CAD build for the part. Positions are in the model's coordinates, mm. A direction names the side the tool comes from. Coordinates: 2 decimals unless noted, no trailing zeros. Order: outer loops, then holes, each group sorted by start corner. A loop starts at its lowest first (then second) coordinate and runs counter-clockwise, first axis right, second up. Notation, with made-up numbers: M -27.75,26 L -7.75,26 A3 ccw -7.75,31 Z; hole C 54.5,17 d4. An arc over 180 degrees is marked long. Write item = value, one per line.
from build123d import *

# Parameters (mm, degrees)
F0_W     = 28.2
F0_H     = 28.2
F0_R     = 11.4
F0_R_2   = 2.25
F1_DEPTH = 28.2
F2_DEPTH = 2
F3_R     = 2.5
F5_D     = 2.5
F5_DEPTH = 5
F5_TIP   = 0.7510757738


with BuildPart() as f1:
    # F0 (on Top) → F1 (new body)
    with BuildSketch(Plane.XY):
        Rectangle(F0_W, F0_H)
        Circle(F0_R, mode=Mode.SUBTRACT)
        Circle(F0_R)
        Circle(F0_R_2, mode=Mode.SUBTRACT)
    extrude(amount=-F1_DEPTH)

    # F0 (on Top) → F2 (join)
    with BuildSketch(Plane.XY):
        Circle(F0_R)
        Circle(F0_R_2, mode=Mode.SUBTRACT)
    extrude(amount=F2_DEPTH)

    # F3
    f3_edges = [f1.edges().sort_by_distance(p)[0] for p in [
        (-14.1, -14.1, -14.1),
        (14.1, -14.1, -14.1),
        (-14.1, 14.1, -14.1),
        (14.1, 14.1, -14.1),
    ]]
    fillet(f3_edges, radius=F3_R)

    # F5
    with Locations(Plane.XY):
        with Locations((-11.5, 11.5), (11.5, 11.5), (11.5, -11.5), (-11.5, -11.5)):
            Hole(F5_D / 2, depth=F5_DEPTH)
            with Locations((0, 0, -(F5_DEPTH + F5_TIP / 2))):  # 118° drill point
                Cone(0, F5_D / 2, F5_TIP, mode=Mode.SUBTRACT)


solid = f1.part
(1) Slice it at B-B, the plane y = 0. Write the cut outline in (x, z), then the cut area to 3 significant figures.
Evaluation:
outline = M -14.1,-28.2 L -2.25,-28.2 L -2.25,2 L -11.4,2 L -11.4,0 L -14.1,0 Z; M 2.25,-28.2 L 14.1,-28.2 L 14.1,0 L 11.4,0 L 11.4,2 L 2.25,2 Z
area = 705 mm²
(2) Tool access for faces 1 (the face through (-0.2, -2.4, 2)), 2 (the face through (12.421, -10.655, -2.535)): list every direction of +Z, -Z, +X, -X, +Y, -Y with a clear straight run to the whole face (end or side of a thin tool).
Evaluation:
face_1 = +Z, +X, -X, +Y, -Y
face_2 = +Z
(3) Slice it at D-D, the plane x = -4.25. Write the cut outline in (y, z).
Evaluation:
outline = M -14.1,-28.2 L 14.1,-28.2 L 14.1,0 L 10.58,0 L 10.58,2 L -10.58,2 L -10.58,0 L -14.1,0 Z
(4) Pull direction X, two halves, no side cores. Call faces 3 (the face through (-13.348, -13.387, -14.297)), 4 (the face through (-3, 0, -28.2)), 5 (the face through (-11.3, 11.42, -5.62)): +X half, -X half, draft (parallel to the pull), parting line (faces both ways), or undercut.
Evaluation:
face_3 = -X half
face_4 = draft
face_5 = undercut
(5) Pin check, flat tips, straight feed: pin 1 Ø7 at (x, y) = (0, 0) entering from +Z; pin 2 Ø2 at (x, y) = (-11.5, 11.5) entering from +Z; pin 3 Ø3 at (x, y) = (11.5, -11.5) entering from +Z. Stop position of each tip, or through.
Evaluation:
pin_1 = 2
pin_2 = -5.15
pin_3 = 0
(6) Wall check: line 1 (Y direction, x = -11.5, z = -2.6); line 2 (Y direction, x = -10.5, z = -1). Give the ranges that are in metal, low to high. Write a range as from..to.
Evaluation:
line_1 = -14.1..-12.75, -10.25..10.25, 12.75..14.1
line_2 = -14.1..-12.25, -10.75..10.75, 12.25..14.1
(7) Slice it at A-A, the plane z = -18. Write the cut outline in (x, y).
Evaluation:
outline = M -14.1,-11.6 A2.5 ccw -11.6,-14.1 L 11.6,-14.1 A2.5 ccw 14.1,-11.6 L 14.1,11.6 A2.5 ccw 11.6,14.1 L -11.6,14.1 A2.5 ccw -14.1,11.6 Z; hole C 0,0 d4.5
(8) Slice it at C-C, the plane y = -5. Write the cut outline in (x, z) (3 decimals), then the cut area to 3 significant figures.
Evaluation:
outline = M -14.1,-28.2 L 14.1,-28.2 L 14.1,0 L 10.245,0 L 10.245,2 L -10.245,2 L -10.245,0 L -14.1,0 Z
area = 836 mm²
